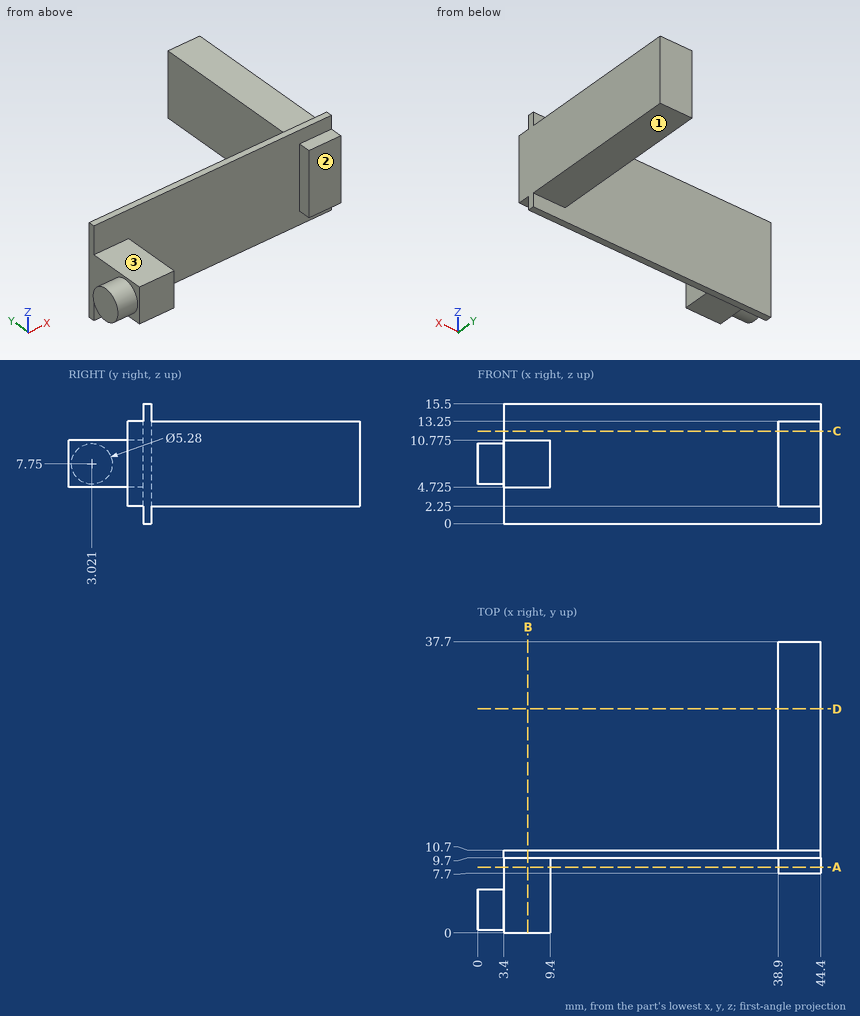
The figure shows three views and two pictorial views of one solid part (mm, origin at its lowest corner). Answer the questions. A direction names the side the tool comes from. Coordinates: 2 decimals unless noted, no trailing zeros. Loops run counter-clockwise (first coordinate to the right, second up) from the corner with the lowest first, then second, coordinate; pieces in that order, holes last.
1) Find section A-A on y = 8.5. Write down the section's boundary in (x, z) (3 decimals).
2) Find the intervals of material crossed by L1, parallel to Z at x = 4, y = 2 (3 decimals); L2, parallel to X at y = 33.5, z = 7; L3, parallel to Y at x = 41, z = 14.5, in increasing order.
3) Find section B-B on x = 6.5. Write down the section's boundary in (y, z) (3 decimals).
4) A tool of negligible diameter and unlimited length cuts with its end or side. For the marked faces 1, 2 and 3, from which of +Z, -Z, +X, -X, +Y, -Y can it reach the whole face along a straight path? Write none if from no direction.
5) Find section C-C on z = 12. Write down the section's boundary in (x, y).
6) Flat-ended cylindrical pins translate along their axes: pin 1 Ø4.5 at (x, y) = (43, 26.5) entering from +Z; pin 2 Ø4.5 at (x, y) = (41, 24.5) entering from -Z; pin 3 Ø3.5 at (y, z) = (19, 8) entering from -X. Find the tip coordinate at first contact, or state that the pin passes through.
7) Find section D-D on y = 29. Write down the section's boundary in (x, z), then the cut area to 3 significant figures.
Values:
1. outline: (3.4, 4.725) - (9.4, 4.725) - (9.4, 10.775) - (3.4, 10.775) - close; (38.9, 2.25) - (44.4, 2.25) - (44.4, 13.25) - (38.9, 13.25) - close
2. L1: z = 4.725 to 10.775
2. L2: x = 38.9 to 44.4
2. L3: y = 9.7 to 10.7
3. outline: (0, 4.725) - (9.7, 4.725) - (9.7, 0) - (10.7, 0) - (10.7, 15.5) - (9.7, 15.5) - (9.7, 10.775) - (0, 10.775) - close
4. face 1: -Z, +X, -X, +Y
4. face 2: +Z, -Z, +X, -Y
4. face 3: +Z, -X, -Y
5. outline: (3.4, 9.7) - (38.9, 9.7) - (38.9, 7.7) - (44.4, 7.7) - (44.4, 37.7) - (38.9, 37.7) - (38.9, 10.7) - (3.4, 10.7) - close
6. pin 1: stops at z = 13.25
6. pin 2: stops at z = 2.25
6. pin 3: stops at x = 38.9
7. outline: (38.9, 2.25) - (44.4, 2.25) - (44.4, 13.25) - (38.9, 13.25) - close
7. area: 60.5 mm2
